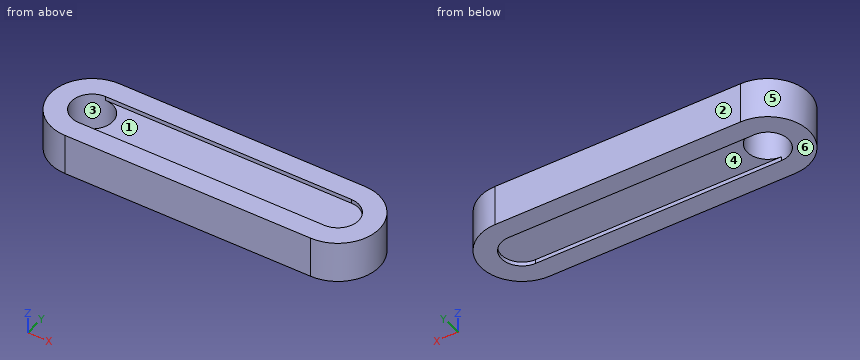
from build123d import *

# Parameters (mm, degrees)
F1_DEPTH = 4
F2_DEPTH = 5


with BuildPart() as f1:
    # F0 (on Top) → F1 (new body, symmetric)
    with BuildSketch(Plane.XY):
        with BuildLine():
            Line((-23.981852, -5), (36.018148, -5))
            ThreePointArc((36.018148, -5), (41.018148, 0), (36.018148, 5))
            Line((36.018148, 5), (-23.981852, 5))
            ThreePointArc((-23.981852, 5), (-18.981852, 0), (-23.981852, -5))
        make_face()
    extrude(amount=F1_DEPTH, both=True)

    # F0 (on Top) → F2 (join, symmetric)
    with BuildSketch(Plane.XY):
        with BuildLine():
            Line((-23.981852, -5), (36.018148, -5))
            ThreePointArc((36.018148, -5), (41.018148, 0), (36.018148, 5))
            Line((36.018148, 5), (-23.981852, 5))
            ThreePointArc((-23.981852, 5), (-18.981852, 0), (-23.981852, -5))
        make_face()
        with BuildLine():
            ThreePointArc((36.018148, -10), (46.018148, 0), (36.018148, 10))
            Line((36.018148, 10), (-23.981852, 10))
            ThreePointArc((-23.981852, 10), (-33.981852, 0), (-23.981852, -10))
            Line((-23.981852, -10), (36.018148, -10))
        make_face()
        with BuildLine():
            ThreePointArc((36.018148, 5), (41.018148, 0), (36.018148, -5))
            Line((36.018148, -5), (-23.981852, -5))
            ThreePointArc((-23.981852, -5), (-28.981852, 0), (-23.981852, 5))
            Line((-23.981852, 5), (36.018148, 5))
        make_face(mode=Mode.SUBTRACT)
    extrude(amount=F2_DEPTH, both=True)


solid = f1.part
The listing builds one solid part. Answer for the finished solid, in the listing's coordinates (mm). Face numbers are marked on the shaded views. A direction names the side the tool comes from. Coordinates: 2 decimals unless noted, no trailing zeros. Loops run counter-clockwise (first coordinate to the right, second up) from the corner with the lowest first, then second, coordinate; pieces in that order, holes last. Notation, with made-up numbers: M 3,30.5 L 25,30.5 A12 ccw 25,48.5 Z; hole C -6.5,41.25 d7. An arc over 180 degrees is marked long. Answer in a Markdown table with one row per item.
1) Determine the mould class of the marked faces 3, 4, 5 and 6 for opening direction Y: released by +Y, released by -Y, zero draft, split by the parting line, or undercut.
Answers below:
| item | result |
|---|---|
| face 3 | undercut |
| face 4 | undercut |
| face 5 | split by the parting line |
| face 6 | zero draft |
2) Given pin 1 (1 mm diameter, centred on x = -18.5, y = -2, fed in from -Z); pin 2 (3 mm diameter, centred on x = 1.5, y = 2, fed in from +Z); pin 3 (4 mm diameter, centred on y = 7.5, z = -3.5, fed in from +X), each flat-ended and moving along its own axis, determine where each tip first touches the part or whether it passes through.
Answers below:
| item | result |
|---|---|
| pin 1 | z = -4 |
| pin 2 | z = 4 |
| pin 3 | x = 44.37 |
3) Find section C-C (z = 1.5). Determine the outline of the cut face in (x, y), then the cut area to 3 significant figures.
Answers below:
| item | result |
|---|---|
| outline | M -23.98,-10 L 36.02,-10 A10 ccw 36.02,10 L -23.98,10 A10 ccw Z; hole C -23.98,0 d10 |
| area | 1,440 mm^2 |
4) Find section B-B (x = 7). Determine the outline of the cut face in (y, z), then the cut area to 3 significant figures.
Answers below:
| item | result |
|---|---|
| outline | M -10,-5 L -5,-5 L -5,-4 L 5,-4 L 5,-5 L 10,-5 L 10,5 L 5,5 L 5,4 L -5,4 L -5,5 L -10,5 Z |
| area | 180 mm^2 |
5) Find section D-D (y = -7.75). Determine the outline of the cut face in (x, z).
Answers below:
| item | result |
|---|---|
| outline | M -30.3,-5 L 42.34,-5 L 42.34,5 L -30.3,5 Z |
6) Find the intervals of material crossed by probe 1 along X at (y, z) = (0, -2.5); probe 2 along Z at (x, y) = (2.5, 0); probe 3 along X at (y, z) = (3.25, -3.75), in increasing order.
Answers below:
| item | result |
|---|---|
| probe 1 | -33.98 to -28.98, -18.98 to 46.02 |
| probe 2 | -4 to 4 |
| probe 3 | -33.44 to -27.78, -20.18 to 45.48 |
7) Which of the six approach directions +Z, -Z, +X, -X, +Y, -Y give full straight-line access (tool end or side, diameter ignored) to the marked faces 1 and 2?
Answers below:
| item | result |
|---|---|
| face 1 | +Z |
| face 2 | +Z, -Z, +X, -X, +Y |
8) Find section A-A (y = 0). Determine the outline of the cut face in (x, z).
Answers below:
| item | result |
|---|---|
| outline | M -33.98,-5 L -28.98,-5 L -28.98,5 L -33.98,5 Z; M -18.98,-4 L 41.02,-4 L 41.02,-5 L 46.02,-5 L 46.02,5 L 41.02,5 L 41.02,4 L -18.98,4 Z |
